Source: CAD feature listing. Evaluate the final solid. Frame: model axes, mm. A direction names the side the tool comes from. Give positions to 0.01 mm unless a question says otherwise; leave off trailing zeros. Loops run counter-clockwise (first coordinate to the right, second up) from the corner with the lowest first, then second, coordinate; pieces in that order, holes last. Notation, with made-up numbers: (55, 37.5) - (81, 37.5) arc R32 cw to (81, 69.5) - close; hole circle Ø11 at (-40, 14). An arc over 180 degrees is marked (long way). Put each result on its own line as item: value.
```python
from build123d import *

# Parameters (mm, degrees)
ESQUISSE1_W      = 80
ESQUISSE1_H      = 80
EXTRUSION1_DEPTH = 53
CONG_1_R         = 5
COQUE1_T         = -2


with BuildPart() as part:
    # Esquisse1 → Extrusion1 (new body)
    with BuildSketch(Plane(origin=(0, 0, 0), x_dir=(1, 0, 0), z_dir=(0, 1, 0))):
        with Locations((40, 40)):
            Rectangle(ESQUISSE1_W, ESQUISSE1_H)
    extrude(amount=EXTRUSION1_DEPTH)

    # Congé1
    cong_1_edges = [part.edges().sort_by_distance(p)[0] for p in [
        (0, 26.5, -80),
        (80, 26.5, -80),
        (80, 26.5, 0),
        (0, 26.5, 0),
    ]]
    fillet(cong_1_edges, radius=CONG_1_R)

    # Coque1
    coque1_openings = [part.faces().sort_by_distance(p)[0] for p in [
        (40, 53, -40),
    ]]
    offset(amount=COQUE1_T, openings=coque1_openings, kind=Kind.INTERSECTION)


solid = part.part
```
1) Mould query, pull axis X, two halves, no side actions, for faces 3 (the cylindrical face through (2.86, 27.86, -2.9)), 4 (the flat face through (40, 26, 0)), 5 (the flat face through (2, 27, -40)), 6 (the cylindrical face through (1, 27, -78)). Classes: pulls with the +X half, pulls with the -X half, needs draft (parallel to the pull), parting line crosses it, or undercut.
Check result:
face 3: undercut
face 4: needs draft
face 5: undercut
face 6: pulls with the -X half
2) Material intervals for line 1 along X through (y, z) = (36.5, -16); line 2 along Z through (x, y) = (41.5, 10.5); line 3 along Y through (x, z) = (71.5, -36), sorted ascending. Write a range as [from, to].
Check result:
line 1: [0, 2], [78, 80]
line 2: [-80, -78], [-2, 0]
line 3: [0, 2]
3) Pin query (flat end, axial travel): P1, Ø23, axis at x = 51.5, z = -30.5, coming from the +Y side. Return the tip coordinate at first contact, or that it passes through.
Check result:
P1: y = 2
4) Access query for faces 1 (the flat face through (39, 0, -41)), 2 (the flat face through (40, 27, -2)). Directions: +Z, -Z, +X, -X, +Y, -Y. A direction counts if a zero-diameter tool reaches every point of the face in a straight line with its end or side. Return the directions, or none.
Check result:
face 1: +Z, -Z, +X, -X, -Y
face 2: +Y
5) Section query A-A, the plane y = 4. Output: boundary loops of the cut face in (x, z), plus the area to 3 significant figures.
Check result:
outline: (0, -75) arc R5 ccw to (5, -80) - (75, -80) arc R5 ccw to (80, -75) - (80, -5) arc R5 ccw to (75, 0) - (5, 0) arc R5 ccw to (0, -5) - close; hole (2, -75) arc R3 ccw to (5, -78) - (75, -78) arc R3 ccw to (78, -75) - (78, -5) arc R3 ccw to (75, -2) - (5, -2) arc R3 ccw to (2, -5) - close
area: 610 mm²
6) Section query B-B, the plane z = -48. Output: boundary loops of the cut face in (x, y).
Check result:
outline: (0, 0) - (80, 0) - (80, 53) - (78, 53) - (78, 2) - (2, 2) - (2, 53) - (0, 53) - close
7) Section query C-C, the plane x = 62. Output: boundary loops of the cut face in (y, z).
Check result:
outline: (0, -80) - (53, -80) - (53, -78) - (2, -78) - (2, -2) - (53, -2) - (53, 0) - (0, 0) - close
